from build123d import *

# Parameters (mm, degrees)
F0_W     = 31.75
F0_H     = 539.75
F1_DEPTH = 19.05
F2_W     = 31.75
F2_H     = 31.75
F3_DEPTH = 9.525
F5_DEPTH = 25.4
F7_DEPTH = 25.4
F9_DEPTH = 25.4


with BuildPart() as f1:
    # F0 (on Right) → F1 (new body)
    with BuildSketch(Plane.YZ):
        Rectangle(F0_W, F0_H)
    extrude(amount=F1_DEPTH)

    # F2 (on face) → F3 (cut)
    with BuildSketch(Plane.YZ.offset(19.05)):
        with Locations((0, 254)):
            Rectangle(F2_W, F2_H)
        with Locations((0, -222.25)):
            Rectangle(F2_W, F2_H)
        with Locations((0, 95.25)):
            Rectangle(F2_W, F2_H)
        with Locations((0, -63.5)):
            Rectangle(F2_W, F2_H)
    extrude(amount=-F3_DEPTH, mode=Mode.SUBTRACT)

    # F4 (on face) → F5 (cut)
    with BuildSketch(Plane.YZ.offset(9.525)):
        with BuildLine():
            ThreePointArc((6.735192, 101.985192), (-6.735192, 101.985192), (-6.735192, 88.514808))
            Line((-6.735192, 88.514808), (6.735192, 101.985192))
        make_face()
        with BuildLine():
            Line((6.735192, 101.985192), (-6.735192, 88.514808))
            ThreePointArc((-6.735192, 88.514808), (3.64506, 86.450047), (9.525, 95.25))
            ThreePointArc((9.525, 95.25), (8.799953, 98.89506), (6.735192, 101.985192))
        make_face()
    extrude(amount=-F5_DEPTH, mode=Mode.SUBTRACT)

    # F6 (on face) → F7 (cut)
    with BuildSketch(Plane.YZ.offset(9.525)):
        with BuildLine():
            ThreePointArc((6.735192, -56.764808), (-6.735192, -56.764808), (-6.735192, -70.235192))
            Line((-6.735192, -70.235192), (6.735192, -56.764808))
        make_face()
        with BuildLine():
            Line((6.735192, -56.764808), (-6.735192, -70.235192))
            ThreePointArc((-6.735192, -70.235192), (3.64506, -72.299953), (9.525, -63.5))
            ThreePointArc((9.525, -63.5), (8.799953, -59.85494), (6.735192, -56.764808))
        make_face()
    extrude(amount=-F7_DEPTH, mode=Mode.SUBTRACT)

    # F8 (on face) → F9 (cut)
    with BuildSketch(Plane.YZ.offset(9.525)):
        with BuildLine():
            ThreePointArc((6.735192, -215.514808), (-6.735192, -215.514808), (-6.735192, -228.985192))
            Line((-6.735192, -228.985192), (6.735192, -215.514808))
        make_face()
        with BuildLine():
            Line((6.735192, -215.514808), (-6.735192, -228.985192))
            ThreePointArc((-6.735192, -228.985192), (3.64506, -231.049953), (9.525, -222.25))
            ThreePointArc((9.525, -222.25), (8.799953, -218.60494), (6.735192, -215.514808))
        make_face()
    extrude(amount=-F9_DEPTH, mode=Mode.SUBTRACT)


solid = f1.part
Work out the finished part from the listing and answer in its coordinate system (mm). A direction names the side the tool comes from. Coordinates: 2 decimals unless noted, no trailing zeros. Write each loop counter-clockwise with the first axis right and the second up, starting at its lowest first coordinate (ties: lowest second). Pieces come first, ordered by that corner, then holes. Notation, with made-up numbers: M -30,-18.5 L -2,-18.5 A21 ccw -2,9.5 Z; hole C 39,32.5 d8. An arc over 180 degrees is marked long. Use one line per item in the form item = value. Start each with the question number.
1. The part is cut by section A-A (x = 13). Give the vertices of the cut face in (y, z) (3 decimals).
2. A tool of negligible diameter and unlimited length cuts with its end or side. For faces 4 (the face through (5, 0, 269.875)), 5 (the face through (14, 0, 111.125)), 6 (the face through (9.525, 0, 254)), from which of +Z, -Z, +X, -X, +Y, -Y can it reach the whole face along a straight path? Write none if from no direction.
3. The mould has two halves that part along Z. Classify faces 1 (the face through (14, 0, -47.625)), 2 (the face through (14, 0, 238.125)), 3 (the face through (0, 0, 4)): released by +Z, released by -Z, zero draft, split by the parting line, or undercut.
4. Each of these flat-tipped pins is pushed along its axis until it touches: P1, Ø10.5, axis at x = 16, y = -7, coming from the +Z side (3 decimals); P2, Ø16, axis at y = 3.5, z = -220.5, coming from the +X side (3 decimals). Where does it stop, or does it pass through?
5. Straight lines are drawn through the part: probe 1 along Z at (x, y) = (13.25, -9.5) (3 decimals); probe 2 along Z at (x, y) = (1.5, -6) (3 decimals); probe 3 along Y at (x, z) = (2.75, -64) (3 decimals). For each, find the intervals that lie inside material, in ascending order. Write a range as from..to.
Evaluation:
q1.outline = M -15.875,-269.875 L 15.875,-269.875 L 15.875,-238.125 L -15.875,-238.125 Z; M -15.875,-206.375 L 15.875,-206.375 L 15.875,-79.375 L -15.875,-79.375 Z; M -15.875,-47.625 L 15.875,-47.625 L 15.875,79.375 L -15.875,79.375 Z; M -15.875,111.125 L 15.875,111.125 L 15.875,238.125 L -15.875,238.125 Z
q2.face_4 = +Z, +X, -X, +Y, -Y
q2.face_5 = +X, +Y, -Y
q2.face_6 = +Z, +X, +Y, -Y
q3.face_1 = undercut
q3.face_2 = released by +Z
q3.face_3 = zero draft
q4.P1 = 238.125
q4.P2 = 9.525
q5.probe_1 = -269.875..-238.125, -206.375..-79.375, -47.625..79.375, 111.125..238.125
q5.probe_2 = -269.875..-229.648, -214.852..-70.898, -56.102..87.852, 102.648..269.875
q5.probe_3 = -15.875..-9.512, 9.512..15.875
